Autodesk Fusion 360 part; units mm, degrees
sketch "Sketch1" plane through (0, 0, 0) normal (0, 0, 1) x (1, 0, 0)
  line L0 (0, 0) -> (8, 0)
  line L1 (8, 0) -> (8, 17)
  line L2 (8, 17) -> (0, 17)
  line L3 (0, 17) -> (0, 0)
  dimension "d1" = 8
  dimension "d2" = 17
extrude "Extrude1" add sketch "Sketch1" along normal blind 3
sketch "Sketch2" plane through (0, 0, 3) normal (0, 0, 1) x (-1, 0, 0)
  line L0 (0, -17) -> (0, 0)
  line L1 (0, 0) -> (-8, 0)
  line L2 (-8, 0) -> (-8, -17)
  line L3 (-8, -17) -> (0, -17)
  line L4 (0, 0) -> (-8, 0)
  line L5 (-8, 0) -> (-8, -4)
  line L6 (-8, -4) -> (0, -4)
  line L7 (0, -4) -> (0, 0)
  dimension "d5" = 8
  dimension "d6" = 4
extrude "Extrude2" add sketch "Sketch2" along normal blind 2 contours L0 L1 L2 L4 L5 L6 L7
sketch "Sketch3" plane through (0, 0, 5) normal (0, 0, 1) x (-1, 0, 0)
  line L0 (0, -4) -> (0, 0)
  line L1 (0, 0) -> (-8, 0)
  line L2 (-8, 0) -> (-8, -4)
  line L3 (-8, -4) -> (0, -4)
  line L4 (0, 0) -> (-8, 0)
  line L5 (-8, 0) -> (-8, -1)
  line L6 (-8, -1) -> (0, -1)
  line L7 (0, -1) -> (0, 0)
  dimension "d9" = 8
extrude "Extrude3" add sketch "Sketch3" along normal blind 3 contours L0 L2 L3 L6
fillet "Fillet1" radius 3 1 edges at (4, 1, 8)
sketch "Sketch4" plane through (0, 0, 3) normal (0, 0, 1) x (-1, 0, 0)
  line L0 (0, -4) -> (-8, -4)
  line L1 (-8, -4) -> (-8, -17)
  line L2 (-8, -17) -> (0, -17)
  line L3 (0, -17) -> (0, -4)
  line L4 (0, -17) -> (-8, -17)
  line L5 (-8, -17) -> (-8, -14)
  line L6 (-8, -14) -> (0, -14)
  line L7 (0, -14) -> (0, -17)
  dimension "d14" = 3
extrude "Extrude4" add sketch "Sketch4" along normal blind 2 contours L1 L2 L3 L4 L5 L6 L7
sketch "Sketch5" plane through (0, 0, 5) normal (0, 0, 1) x (-1, 0, 0)
  line L0 (0, -14) -> (-8, -14)
  line L1 (-8, -14) -> (-8, -17)
  line L2 (-8, -17) -> (0, -17)
  line L3 (0, -17) -> (0, -14)
  line L4 (-8, -17) -> (-6, -17)
  line L5 (-6, -17) -> (-6, -14)
  line L6 (-6, -14) -> (-8, -14)
  line L7 (-8, -14) -> (-8, -17)
  line L8 (0, -17) -> (-2, -17)
  line L9 (-2, -17) -> (-2, -14)
  line L10 (-2, -14) -> (0, -14)
  line L11 (0, -14) -> (0, -17)
  dimension "d17" = 2
  dimension "d18" = 2
extrude "Extrude5" add sketch "Sketch5" along normal blind 2 contours L0 L2 L5 L9
fillet "Fillet2" radius 2 2 edges at (2, 15.5, 7) (6, 15.5, 7)
sketch "Sketch6" plane through (0, 0, 0) normal (0, -1, 0) x (1, 0, 0)
  line L0 (0, 0) -> (8, 0)
  line L1 (8, 0) -> (8, 5)
  line L2 (8, 5) -> (0, 5)
  line L3 (0, 5) -> (0, 0)
  line L4 (0, 0) -> (2, 0)
  line L5 (2, 0) -> (2, 2)
  line L6 (2, 2) -> (0, 2)
  line L7 (0, 2) -> (0, 0)
  line L8 (8, 0) -> (6, 0)
  line L9 (6, 0) -> (6, 2)
  line L10 (6, 2) -> (8, 2)
  line L11 (8, 2) -> (8, 0)
  line L12 (2, 2) -> (6, 2)
  line L13 (6, 2) -> (6, 0)
  line L14 (6, 0) -> (2, 0)
  line L15 (2, 0) -> (2, 2)
  dimension "d23" = 2
  dimension "d24" = 2
  dimension "d25" = 2
extrude "Extrude6" cut sketch "Sketch6" against normal blind 23 contours L0 L5 L9 L12 L13 L14 L15
sketch "Sketch7" plane through (0, 0, 3) normal (0, 0, 1) x (-1, 0, 0)
  line L0 (-8, -14) -> (0, -14)
  line L1 (0, -14) -> (0, -4)
  line L2 (0, -4) -> (-8, -4)
  line L3 (-8, -4) -> (-8, -14)
  line L4 (0, -4) -> (-3, -4)
  line L5 (-3, -4) -> (-3, -14)
  line L6 (-3, -14) -> (0, -14)
  line L7 (0, -14) -> (0, -4)
  line L8 (-8, -4) -> (-5, -4)
  line L9 (-5, -4) -> (-5, -14)
  line L10 (-5, -14) -> (-8, -14)
  line L11 (-8, -14) -> (-8, -4)
  dimension "d28" = 3
  dimension "d29" = 3
extrude "Extrude7" add sketch "Sketch7" along normal blind 1 contours L0 L2 L5 L9
sketch "Sketch8" plane through (0, 0, 2) normal (0, 0, -1) x (1, 0, 0)
  line L0 (2, -17) -> (6, -17)
  line L1 (6, -17) -> (6, 0)
  line L2 (6, 0) -> (2, 0)
  line L3 (2, 0) -> (2, -17)
  line L4 (6, 0) -> (2, 0)
  line L5 (2, 0) -> (2, -4)
  line L6 (2, -4) -> (6, -4)
  line L7 (6, -4) -> (6, 0)
  line L8 (6, 0) -> (5, 0)
  line L9 (5, 0) -> (5, -4)
  line L10 (5, -4) -> (6, -4)
  line L11 (6, -4) -> (6, 0)
  line L12 (2, 0) -> (3, 0)
  line L13 (3, 0) -> (3, -4)
  line L14 (3, -4) -> (2, -4)
  line L15 (2, -4) -> (2, 0)
  line L16 (6, -17) -> (2, -17)
  line L17 (2, -17) -> (2, -14)
  line L18 (2, -14) -> (6, -14)
  line L19 (6, -14) -> (6, -17)
  line L20 (6, -17) -> (5, -17)
  line L21 (5, -17) -> (5, -14)
  line L22 (5, -14) -> (6, -14)
  line L23 (6, -14) -> (6, -17)
  line L24 (2, -17) -> (3, -17)
  line L25 (3, -17) -> (3, -14)
  line L26 (3, -14) -> (2, -14)
  line L27 (2, -14) -> (2, -17)
  dimension "d32" = 4
  dimension "d33" = 1
  dimension "d34" = 1
  dimension "d35" = 3
  dimension "d36" = 1
  dimension "d37" = 1
extrude "Extrude8" cut sketch "Sketch8" against normal blind 2 contours L0 L16 L18 L21 L25 | L2 L4 L6 L9 L13
Check sheet for the modelled part. Datum: model origin and axes. Units: mm. A direction names the side the tool comes from. Round coordinates to 2 decimals unless told otherwise and drop trailing zeros. Order: outer loops, then holes, each group sorted by start corner. A loop starts at its lowest first (then second) coordinate and runs counter-clockwise, first axis right, second up. Notation, with made-up numbers: (25.5, 29) -> (60.5, 29) arc R21 ccw to (60.5, 38) -> close; hole circle Ø3 at (-3.5, 69). An arc over 180 degrees is marked (long way). Use CSV: the item, a comma, the result in double quotes.
(1) Cross-section at B-B (z = 4.25). Record the boundary of the cut face in (x, y).
Worked out:
outline,"(0, 0) -> (8, 0) -> (8, 4) -> (0, 4) -> close; (0, 14) -> (8, 14) -> (8, 17) -> (0, 17) -> close"
(2) Cross-section at C-C (y = 12). Record the boundary of the cut face in (x, z).
Worked out:
outline,"(0, 0) -> (2, 0) -> (2, 2) -> (6, 2) -> (6, 0) -> (8, 0) -> (8, 3) -> (5, 3) -> (5, 4) -> (3, 4) -> (3, 3) -> (0, 3) -> close"
(3) Tool access check on faces 4 (the face through (7, 15, 5)), 5 (the face through (4, 14, 3)), 6 (the face through (4, 2, 4)), 7 (the face through (4.1, 0.5, 5)), 8 (the face through (6, 9, 3)). Record the directions out of +Z, -Z, +X, -X, +Y, -Y that give a thin tool (end or side, any length) a straight path to the whole face; none if there is none.
Worked out:
face 4,"+Z, +X, +Y"
face 5,"-Z, +Y"
face 6,"-Z, -Y"
face 7,"+Z, +X, -X, -Y"
face 8,"+Z, +X"
(4) Material ranges on line 1 along Y through (x, z) = (4, 4.5); line 2 along Z through (x, y) = (5.25, 13.25); line 3 along X through (y, z) = (7, 0.5), recorded low to high. Write a range as from..to.
Worked out:
line 1,"0..4, 14..17"
line 2,"2..3"
line 3,"0..2, 6..8"
(5) Depth check by flat-ended pin: pin 1 (0.6 mm diameter, centred on x = 4, z = 3.5, fed in from -Y); pin 2 (3.5 mm diameter, centred on x = 6.5, y = 8, fed in from +Z); pin 3 (4 mm diameter, centred on x = 2, y = 12.5, fed in from +Z); pin 4 (2 mm diameter, centred on y = 9, z = 5.5, fed in from -X). Enter the tip coordinate at first touch or a pass-through.
Worked out:
pin 1,"y = 4"
pin 2,"z = 4"
pin 3,"z = 6.88"
pin 4,"through"
(6) Draft check along X on faces 1 (the face through (2, 8, 1)), 2 (the face through (3, 8.9, 3.5)), 3 (the face through (6, 0, 3)). Enter one of: pulls with the +X half, pulls with the -X half, needs draft (parallel to the pull), parting line crosses it, or undercut.
Worked out:
face 1,"undercut"
face 2,"pulls with the -X half"
face 3,"needs draft"
